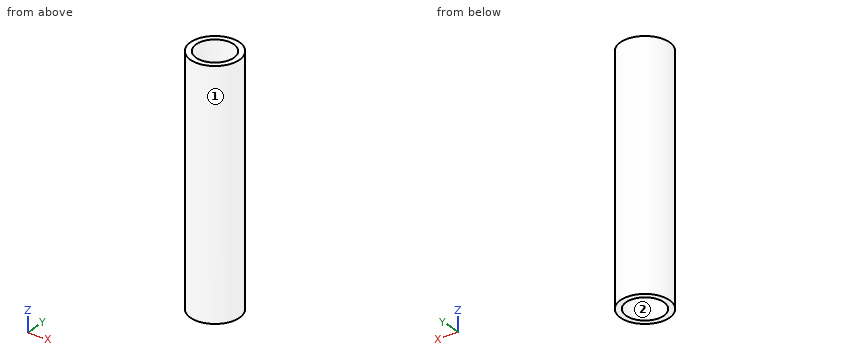
from build123d import *

# Parameters (mm, degrees)
EXTRUDE1_DEPTH                  = 19.2
EXTRUDE1_DEPTH_BACK             = 19.2
SKETCH1_R                       = 3.9
M6X1_0_TAPPED_HOLE3_D           = 5
M6X1_0_TAPPED_HOLE3_DEPTH       = 15
M6X1_0_TAPPED_HOLE3_CBORE_D     = 6
M6X1_0_TAPPED_HOLE3_CBORE_DEPTH = 12
M6X1_0_TAPPED_HOLE3_TIP         = 1.502151548
M6X1_0_TAPPED_HOLE4_D           = 5
M6X1_0_TAPPED_HOLE4_DEPTH       = 15
M6X1_0_TAPPED_HOLE4_CBORE_D     = 6
M6X1_0_TAPPED_HOLE4_CBORE_DEPTH = 12
M6X1_0_TAPPED_HOLE4_TIP         = 1.502151548


with BuildPart() as part:
    # Sketch1 → Extrude1 (new, two sides: drawn at the far end of the back side and taken through both)
    with BuildSketch(Plane.XY.offset(-EXTRUDE1_DEPTH_BACK)):
        with Locations(Location((12.965088215, 18.997538987, 0), (0, 0, 90))):
            Circle(SKETCH1_R)
    extrude(amount=EXTRUDE1_DEPTH + EXTRUDE1_DEPTH_BACK)

    # M6x1.0 Tapped Hole3
    with Locations(Plane(origin=(12.965088215, 18.997538987, 19.2), x_dir=(0, 1, 0), z_dir=(0, 0, 1))):
        with Locations((0, 0)):
            CounterBoreHole(M6X1_0_TAPPED_HOLE3_D / 2, M6X1_0_TAPPED_HOLE3_CBORE_D / 2, M6X1_0_TAPPED_HOLE3_CBORE_DEPTH, depth=M6X1_0_TAPPED_HOLE3_DEPTH)
            with Locations((0, 0, -(M6X1_0_TAPPED_HOLE3_DEPTH + M6X1_0_TAPPED_HOLE3_TIP / 2))):  # 118° drill point
                Cone(0, M6X1_0_TAPPED_HOLE3_D / 2, M6X1_0_TAPPED_HOLE3_TIP, mode=Mode.SUBTRACT)

    # M6x1.0 Tapped Hole4
    with Locations(Plane(origin=(12.965088215, 18.997538987, -19.2), x_dir=(0, -1, 0), z_dir=(0, 0, -1))):
        with Locations((0, 0)):
            CounterBoreHole(M6X1_0_TAPPED_HOLE4_D / 2, M6X1_0_TAPPED_HOLE4_CBORE_D / 2, M6X1_0_TAPPED_HOLE4_CBORE_DEPTH, depth=M6X1_0_TAPPED_HOLE4_DEPTH)
            with Locations((0, 0, -(M6X1_0_TAPPED_HOLE4_DEPTH + M6X1_0_TAPPED_HOLE4_TIP / 2))):  # 118° drill point
                Cone(0, M6X1_0_TAPPED_HOLE4_D / 2, M6X1_0_TAPPED_HOLE4_TIP, mode=Mode.SUBTRACT)


solid = part.part
Model file for the job. Use its own axes, mm. Face numbers are marked on the shaded views. Coordinates: 2 decimals unless noted, no trailing zeros. Order: outer loops, then holes, each group sorted by start corner. A loop starts at its lowest first (then second) coordinate and runs counter-clockwise, first axis right, second up. Notation, with made-up numbers: M 27,77.25 L 83,77.25 A9 ccw 83,86.25 Z; hole C -22,66 d4. An arc over 180 degrees is marked long. Return JSON: item names as keys, results as strings.
1. Pull direction X, two halves, no side cores. Call the marked faces 1 and 2: +X half, -X half, draft (parallel to the pull), parting line (faces both ways), or undercut.
Ans:
{"face 1": "parting line", "face 2": "undercut"}
2. Flat gauge pins, fed straight in: pin 1 (1.8 mm diameter, centred on x = 12.5, y = 20, fed in from -Z); pin 2 (3.5 mm diameter, centred on x = 12.97, y = 19, fed in from -Z); pin 3 (1 mm diameter, centred on x = 12, y = 17, fed in from -Z). Where does each tip first touch, or does it go through?
Ans:
{"pin 1": "z = -3.9", "pin 2": "z = -3.75", "pin 3": "z = -7.2"}
3. Drill centre lines: probe 1 along Y at (x, z) = (13, 13.5); probe 2 along Y at (x, z) = (13.5, 9); probe 3 along X at (y, z) = (20.25, -5.5). Where is each one in solid material? Low to high.
Ans:
{"probe 1": "15.1 to 16, 22 to 22.9", "probe 2": "15.13 to 16.05, 21.95 to 22.86", "probe 3": "9.27 to 10.8, 15.13 to 16.66"}
4. Saw through at A-A (z = -5.5). Give the cut face in (x, y).
Ans:
{"outline": "C 12.97,19 d7.8; hole C 12.97,19 d5"}
5. Saw through at C-C (z = -15). Give the cut face in (x, y).
Ans:
{"outline": "C 12.97,19 d7.8; hole C 12.97,19 d6"}
6. Saw through at B-B (z = 2). Give the cut face in (x, y), and give its area (3 significant figures).
Ans:
{"outline": "C 12.97,19 d7.8", "area": "47.8 mm^2"}
